from build123d import *

# Parameters (mm, degrees)
F0_R     = 6
F0_R_2   = 1.5
F1_DEPTH = 15
F2_R     = 6
F2_R_2   = 4
F3_DEPTH = 10
F6_ANGLE = 90


with BuildPart() as f1:
    # F0 (on Top) → F1 (new body)
    with BuildSketch(Plane.XY):
        Circle(F0_R)
        Circle(F0_R_2, mode=Mode.SUBTRACT)
    extrude(amount=F1_DEPTH)

    # F2 (on Right) → F3 (join)
    with BuildSketch(Plane.YZ):
        Circle(F2_R)
        Circle(F2_R_2, mode=Mode.SUBTRACT)
    extrude(amount=F3_DEPTH)

    # F4 (on face) → F6 (revolve)
    with BuildSketch(Plane(origin=(0, 0, 0), x_dir=(1, 0, 0), z_dir=(0, 0, -1))):
        with BuildLine():
            Line((0, -6), (0, 6))
            ThreePointArc((0, 6), (-6, 0), (0, -6))
        make_face()
    revolve(axis=Axis((0, -1.910034, 0), (0, -1, 0)), revolution_arc=F6_ANGLE)


solid = f1.part
Input: part model. Units: mm. Frame: model coordinates. A direction names the side the tool comes from. Round coordinates to 2 decimals unless told otherwise and drop trailing zeros. Loops run counter-clockwise (first coordinate to the right, second up) from the corner with the lowest first, then second, coordinate; pieces in that order, holes last. Notation, with made-up numbers: (13.5, 28.25) -> (19.5, 28.25) arc R26 cw to (19.5, 53.25) -> close; hole circle Ø2 at (71.25, 42). An arc over 180 degrees is marked (long way). Answer as a JSON object with one key per item and string values. Group by question number.
1) Draft query along X for faces 1 (the cylindrical face through (-1.5, 0.07, 7.4)), 2 (the flat face through (10, -1.42, -3.92)), 3 (the cylindrical face through (-6, 0, 7)). Return one class per face: +X half, -X half, draft (parallel to the pull), parting line (faces both ways), or undercut.
2) Section query D-D on y = -1.75. Output: boundary loops of the cut face in (x, z), plus the area to 3 significant figures.
3) Section query A-A on y = 0. Output: boundary loops of the cut face in (x, z).
4) Section query C-C on x = 7.75. Output: boundary loops of the cut face in (y, z).
5) Pin query (flat end, axial travel): pin 1 (6.5 mm diameter, centred on y = 0, z = 0, fed in from +X); pin 2 (2 mm diameter, centred on y = -1, z = -1.5, fed in from +X); pin 3 (3 mm diameter, centred on x = -1.5, y = 3.5, fed in from -Z). Return the tip coordinate at first contact, or that it passes through.
6) Reachability of faces 4 (the flat face through (1.2, -1.2, 15)), 5 (the cylindrical face through (6.041, -0.867, -3.905)), 6 (the cylindrical face through (1, 0, 4)), 7 (the flat face through (0, 0, 5)) from +Z, -Z, +X, -X, +Y, -Y: full face, straight path, thin tool, end or side. Return the list, or none.
7) Ray query, L1, parallel to X at y = 0, z = 3; L2, parallel to Z at x = 2.5, y = 0; L3, parallel to Z at x = 5.25, y = -3.5. Return the intervals inside material, ascending.
8) Section query B-B on z = 2.25. Output: boundary loops of the cut face in (x, y).
Reply:
{
 "1": {"face 1": "undercut", "face 2": "+X half", "face 3": "parting line"},
 "2": {"outline": "(-5.74, 0) arc R5.74 ccw to (0, -5.74) -> (10, -5.74) -> (10, -3.6) -> (0, -3.6) -> (0, 0) -> (5.74, 0) -> (5.74, 3.6) -> (10, 3.6) -> (10, 5.74) -> (5.74, 5.74) -> (5.74, 15) -> (-5.74, 15) -> close", "area": "229 mm2"},
 "3": {"outline": "(-6, 0) arc R6 ccw to (0, -6) -> (10, -6) -> (10, -4) -> (0, -4) -> (0, 0) -> (-1.5, 0) -> (-1.5, 15) -> (-6, 15) -> close; (0, 4) -> (1.5, 4) -> (1.5, 0) -> (6, 0) -> (6, 4) -> (10, 4) -> (10, 6) -> (6, 6) -> (6, 15) -> (1.5, 15) -> (1.5, 6) -> (0, 6) -> close"},
 "4": {"outline": "circle Ø12 at (0, 0); hole circle Ø8 at (0, 0)"},
 "5": {"pin 1": "stops at x = 6", "pin 2": "stops at x = 0", "pin 3": "stops at z = -5.54"},
 "6": {"face 4": "+Z, +X, -X, +Y, -Y", "face 5": "+X", "face 6": "none", "face 7": "+Z"},
 "7": {"L1": "x = -6 to -1.5, 1.5 to 6", "L2": "z = -6 to -4, 0 to 15", "L3": "z = -4.87 to -1.94, 1.94 to 4.87"},
 "8": {"outline": "(2.25, -5.56) -> (10, -5.56) -> (10, -3.31) -> (5.01, -3.31) arc R6 ccw to (5.01, 3.31) -> (10, 3.31) -> (10, 5.56) -> (2.25, 5.56) arc R6 ccw (long way) to start; hole circle Ø3 at (0, 0)"}
}
